```python
from build123d import *

# Parameters (mm, degrees)
BOSS_EXTRUDE1_DEPTH = 101.6


with BuildPart() as part:
    # Sketch1 → Boss-Extrude1 (new body)
    with BuildSketch(Plane(origin=(0, 0, -302.26), x_dir=(-1, 0, 0), z_dir=(0, 0, -1))):
        with BuildLine():
            Line((2.286, 7.60119137), (2.286, 5.69619137))
            ThreePointArc((2.286, 5.69619137), (2.100012806, 5.247178564), (1.651, 5.06119137))
            Line((1.651, 5.06119137), (-1.651, 5.06119137))
            ThreePointArc((-1.651, 5.06119137), (-2.100012806, 5.247178564), (-2.286, 5.69619137))
            Line((-2.286, 5.69619137), (-2.286, 7.60119137))
            ThreePointArc((-2.286, 7.60119137), (0, -7.9375), (2.286, 7.60119137))
        make_face()
    extrude(amount=-BOSS_EXTRUDE1_DEPTH)


solid = part.part
```
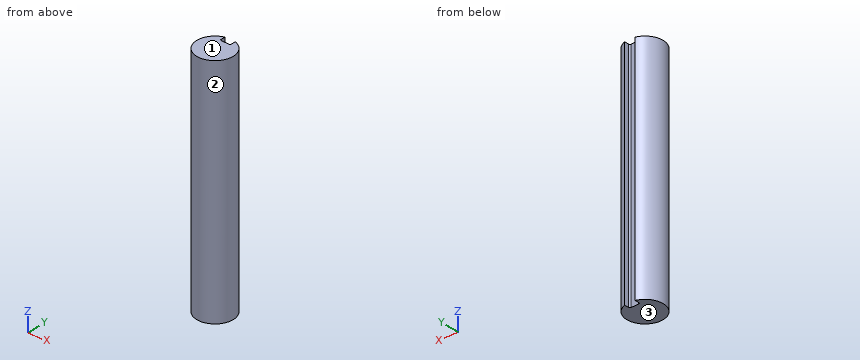
Source: CAD feature listing. Evaluate the final solid. Frame: model axes, mm. Face numbers are marked on the shaded views. Coordinates: 2 decimals unless noted, no trailing zeros. Write each loop counter-clockwise with the first axis right and the second up, starting at its lowest first coordinate (ties: lowest second). Pieces come first, ordered by that corner, then holes. Notation, with made-up numbers: (-20.75, 85.25) -> (3.25, 85.25) arc R19 ccw to (3.25, 119.25) -> close; hole circle Ø8 at (30, -32). An arc over 180 degrees is marked (long way). Return JSON: item names as keys, results as strings. Group by question number.
1) Contact query for flat-ended pins moving along their axis: P1, Ø6, axis at x = 6, z = -257, coming from the +Y side; P2, Ø0.6, axis at y = 6.5, z = -261, coming from the +X side; P3, Ø5, axis at y = 4.5, z = -268, coming from the -X side. Output: stop coordinate, or through.
2) Section query C-C, the plane y = -6.5. Return loops of the section in (x, z), plus the area to 3 significant figures.
3) Mould query, pull axis Z, two halves, no side actions, for the marked faces 1, 2 and 3. Classes: +Z half, -Z half, draft (parallel to the pull), parting line (faces both ways), or undercut.
4) Section query B-B, the plane x = 0. Return loops of the section in (y, z).
5) Section query A-A, the plane z = -252. Return loops of the section in (x, y) (1 decimal), plus the area to 3 significant figures.
6) Ray query, line 1 along Y through (x, z) = (-0.5, -245); line 2 along X through (y, z) = (5.25, -225); line 3 along X through (y, z) = (6, -263). Return the intervals inside material, ascending.
From the geometry:
{
 "1": {"P1": "y = 7.35", "P2": "x = 4.96", "P3": "x = -7.68"},
 "2": {"outline": "(-4.56, -302.26) -> (4.56, -302.26) -> (4.56, -200.66) -> (-4.56, -200.66) -> close", "area": "926 mm²"},
 "3": {"face 1": "+Z half", "face 2": "draft", "face 3": "-Z half"},
 "4": {"outline": "(-7.94, -302.26) -> (5.06, -302.26) -> (5.06, -200.66) -> (-7.94, -200.66) -> close"},
 "5": {"outline": "(-2.3, 5.7) -> (-2.3, 7.6) arc R7.9 ccw (long way) to (2.3, 7.6) -> (2.3, 5.7) arc R0.6 cw to (1.7, 5.1) -> (-1.7, 5.1) arc R0.6 cw to start", "area": "185 mm²"},
 "6": {"line 1": "-7.92 to 5.06", "line 2": "-5.95 to -2.1, 2.1 to 5.95", "line 3": "-5.2 to -2.29, 2.29 to 5.2"}
}
